The model under review builds one solid part; all positions refer to its coordinate system, in mm. A direction names the side the tool comes from. Round coordinates to 2 decimals unless told otherwise and drop trailing zeros. Loops run counter-clockwise (first coordinate to the right, second up) from the corner with the lowest first, then second, coordinate; pieces in that order, holes last. Notation, with made-up numbers: (3.5, 85.25) - (42.5, 85.25) arc R18 cw to (42.5, 109.25) - close; hole circle Ø3 at (-34, 13). An arc over 180 degrees is marked (long way). Answer as CSV lines item,"result".
from build123d import *

# Parameters (mm, degrees)
SKETCH2_W           = 86.9
SKETCH2_H           = 57
SKETCH2_W_2         = 86.5
SKETCH2_H_2         = 56.6
SKETCH2_W_3         = 75.7
SKETCH2_H_3         = 51.1
BOSS_EXTRUDE2_DEPTH = 1.5
SKETCH2_3_W         = 96.4
SKETCH2_3_H         = 63
SKETCH2_3_W_2       = 86.9
SKETCH2_3_H_2       = 57
BOSS_EXTRUDE3_DEPTH = 27
CHAMFER1_SIZE       = 1
SKETCH3_W           = 96.4
SKETCH3_H           = 63
SKETCH3_W_2         = 93.4
SKETCH3_H_2         = 60
BOSS_EXTRUDE4_DEPTH = 1.5
CHAMFER2_SIZE       = 1.5
SKETCH6_W           = 9.728035046
SKETCH6_H           = 14
CUT_EXTRUDE1_DEPTH  = 6
SKETCH10_W          = 3
SKETCH10_H          = 37.1
CUT_EXTRUDE2_DEPTH  = 23.4
SKETCH11_W          = 3.109966679
SKETCH11_H          = 18.3
CUT_EXTRUDE6_DEPTH  = 20.1
SKETCH12_W          = 13.8
SKETCH12_H          = 3.233091644
CUT_EXTRUDE7_DEPTH  = 10
SKETCH13_W          = 20.000720153
SKETCH13_H          = 4.04568645
CUT_EXTRUDE8_DEPTH  = 14
SKETCH15_W          = 10.8
SKETCH15_H          = 3.606090768
CUT_EXTRUDE9_DEPTH  = 13.4
CHAMFER3_SIZE       = 1.5
CHAMFER4_SIZE       = 1.5
CHAMFER5_SIZE       = 1.5
CHAMFER6_SIZE       = 1.5
CHAMFER7_SIZE       = 1.5
CUT_EXTRUDE11_DEPTH = 4
CUT_EXTRUDE12_DEPTH = 8
SKETCH19_R          = 3.5
CUT_EXTRUDE13_DEPTH = 10
CUT_EXTRUDE14_DEPTH = 4.8


with BuildPart() as part:
    # Sketch2 → Boss-Extrude2 (new body)
    # profile 1 of 2: a face of its own
    with BuildSketch(Plane(origin=(0, 0, 0), x_dir=(0, 0, -1), z_dir=(1, 0, 0))):
        with Locations((-2.142915598, 3.029012225)):
            Rectangle(SKETCH2_W, SKETCH2_H)
        with Locations((-2.142915598, 3.029012225)):
            Rectangle(SKETCH2_W_2, SKETCH2_H_2, mode=Mode.SUBTRACT)
    # profile 2 of 2: a face of its own
    with BuildSketch(Plane(origin=(0, 0, 0), x_dir=(0, 0, -1), z_dir=(1, 0, 0))):
        with Locations((-2.142915598, 3.029012225)):
            Rectangle(SKETCH2_W_2, SKETCH2_H_2)
        with Locations((-0.142915598, 3.279012225)):
            Rectangle(SKETCH2_W_3, SKETCH2_H_3, mode=Mode.SUBTRACT)
    extrude(amount=-BOSS_EXTRUDE2_DEPTH)

    # Sketch2_3 → Boss-Extrude3 (add)
    with BuildSketch(Plane(origin=(0, 0, 0), x_dir=(0, 0, -1), z_dir=(1, 0, 0))):
        with Locations((-0.392915598, 3.029012225)):
            Rectangle(SKETCH2_3_W, SKETCH2_3_H)
        with Locations((-2.142915598, 3.029012225)):
            Rectangle(SKETCH2_3_W_2, SKETCH2_3_H_2, mode=Mode.SUBTRACT)
    extrude(amount=-BOSS_EXTRUDE3_DEPTH)

    # Chamfer1
    chamfer1_edges = [part.edges().sort_by_distance(p)[0] for p in [
        (-0.75, 28.829012225, 37.992915598),
        (-0.75, -22.270987775, 37.992915598),
        (-0.75, -22.270987775, -37.707084402),
        (-0.75, 28.829012225, -37.707084402),
    ]]
    chamfer(chamfer1_edges, length=CHAMFER1_SIZE)

    # Sketch3 → Boss-Extrude4 (add)
    with BuildSketch(Plane.ZY.offset(27)):
        with Locations((0.392915598, 3.029012225)):
            Rectangle(SKETCH3_W, SKETCH3_H)
        with Locations((0.392915598, 3.029012225)):
            Rectangle(SKETCH3_W_2, SKETCH3_H_2, mode=Mode.SUBTRACT)
    extrude(amount=BOSS_EXTRUDE4_DEPTH)

    # Chamfer2
    chamfer2_edges = [part.edges().sort_by_distance(p)[0] for p in [
        (-14.25, 34.529012225, -47.807084402),
        (-14.25, -28.470987775, -47.807084402),
        (-14.25, -28.470987775, 48.592915598),
        (-14.25, 34.529012225, 48.592915598),
    ]]
    chamfer(chamfer2_edges, length=CHAMFER2_SIZE)

    # Sketch6 → Cut-Extrude1 (cut)
    with BuildSketch(Plane.ZY.offset(28.5)):
        with Locations((-46.171101925, 2.829012225)):
            Rectangle(SKETCH6_W, SKETCH6_H)
    extrude(amount=-CUT_EXTRUDE1_DEPTH, mode=Mode.SUBTRACT)

    # Sketch10 → Cut-Extrude2 (cut)
    with BuildSketch(Plane.ZY.offset(28.5)):
        with Locations((47.092915598, -6.920987775)):
            Rectangle(SKETCH10_W, SKETCH10_H)
    extrude(amount=-CUT_EXTRUDE2_DEPTH, mode=Mode.SUBTRACT)

    # Sketch11 → Cut-Extrude6 (cut)
    with BuildSketch(Plane.ZY.offset(28.5)):
        with Locations((47.037932259, 20.779012225)):
            Rectangle(SKETCH11_W, SKETCH11_H)
    extrude(amount=-CUT_EXTRUDE6_DEPTH, mode=Mode.SUBTRACT)

    # Sketch12 → Cut-Extrude7 (cut)
    with BuildSketch(Plane.ZY.offset(28.5)):
        with Locations((-30.410119612, 32.912466403)):
            Rectangle(SKETCH12_W, SKETCH12_H)
    extrude(amount=-CUT_EXTRUDE7_DEPTH, mode=Mode.SUBTRACT)

    # Sketch13 → Cut-Extrude8 (cut)
    with BuildSketch(Plane.ZY.offset(28.5)):
        with Locations((-9.312541512, 33.035392559)):
            Rectangle(SKETCH13_W, SKETCH13_H)
    extrude(amount=-CUT_EXTRUDE8_DEPTH, mode=Mode.SUBTRACT)

    # Sketch15 → Cut-Extrude9 (cut)
    with BuildSketch(Plane.ZY.offset(28.5)):
        with Locations((12.393292701, 33.319062827)):
            Rectangle(SKETCH15_W, SKETCH15_H)
    extrude(amount=-CUT_EXTRUDE9_DEPTH, mode=Mode.SUBTRACT)

    # Chamfer3
    chamfer3_edges = [part.edges().sort_by_distance(p)[0] for p in [
        (-18.5, 33.029012225, -37.310119612),
        (-18.5, 33.029012225, -23.510119612),
    ]]
    chamfer(chamfer3_edges, length=CHAMFER3_SIZE)

    # Chamfer4
    chamfer4_edges = [part.edges().sort_by_distance(p)[0] for p in [
        (-14.5, 33.029012225, -19.312901588),
        (-14.5, 33.029012225, 0.687818565),
    ]]
    chamfer(chamfer4_edges, length=CHAMFER4_SIZE)

    # Chamfer5
    chamfer5_edges = [part.edges().sort_by_distance(p)[0] for p in [
        (-15.1, 33.029012225, 6.993292701),
        (-15.1, 33.029012225, 17.793292701),
    ]]
    chamfer(chamfer5_edges, length=CHAMFER5_SIZE)

    # Chamfer6
    chamfer6_edges = [part.edges().sort_by_distance(p)[0] for p in [
        (-22.5, -4.170987775, -44.557084402),
        (-22.5, 9.829012225, -44.557084402),
    ]]
    chamfer(chamfer6_edges, length=CHAMFER6_SIZE)

    # Chamfer7
    chamfer7_edges = [part.edges().sort_by_distance(p)[0] for p in [
        (-5.1, 11.629012225, 47.092915598),
        (-5.1, -25.470987775, 47.092915598),
    ]]
    chamfer(chamfer7_edges, length=CHAMFER7_SIZE)

    # Sketch17 → Cut-Extrude11 (cut)
    with BuildSketch(Plane.XZ.offset(28.470987775)):
        with BuildLine():
            Line((-20.830033603, 35.662637039), (-7.669966397, 35.662637039))
            ThreePointArc((-7.669966397, 35.662637039), (-6.419966397, 34.412637039), (-7.669966397, 33.162637039))
            Line((-7.669966397, 33.162637039), (-20.830033603, 33.162637039))
            ThreePointArc((-20.830033603, 33.162637039), (-22.080033603, 34.412637039), (-20.830033603, 35.662637039))
        make_face()
        with BuildLine():
            Line((-20.830033603, 29.962637039), (-7.669966397, 29.962637039))
            ThreePointArc((-7.669966397, 29.962637039), (-6.419966397, 28.712637039), (-7.669966397, 27.462637039))
            Line((-7.669966397, 27.462637039), (-20.830033603, 27.462637039))
            ThreePointArc((-20.830033603, 27.462637039), (-22.080033603, 28.712637039), (-20.830033603, 29.962637039))
        make_face()
        with BuildLine():
            Line((-20.830033603, 24.262637039), (-7.669966397, 24.262637039))
            ThreePointArc((-7.669966397, 24.262637039), (-6.419966397, 23.012637039), (-7.669966397, 21.762637039))
            Line((-7.669966397, 21.762637039), (-20.830033603, 21.762637039))
            ThreePointArc((-20.830033603, 21.762637039), (-22.080033603, 23.012637039), (-20.830033603, 24.262637039))
        make_face()
        with BuildLine():
            Line((-20.830033603, 18.562637039), (-7.669966397, 18.562637039))
            ThreePointArc((-7.669966397, 18.562637039), (-6.419966397, 17.312637039), (-7.669966397, 16.062637039))
            Line((-7.669966397, 16.062637039), (-20.830033603, 16.062637039))
            ThreePointArc((-20.830033603, 16.062637039), (-22.080033603, 17.312637039), (-20.830033603, 18.562637039))
        make_face()
        with BuildLine():
            Line((-20.830033603, 12.862637039), (-7.669966397, 12.862637039))
            ThreePointArc((-7.669966397, 12.862637039), (-6.419966397, 11.612637039), (-7.669966397, 10.362637039))
            Line((-7.669966397, 10.362637039), (-20.830033603, 10.362637039))
            ThreePointArc((-20.830033603, 10.362637039), (-22.080033603, 11.612637039), (-20.830033603, 12.862637039))
        make_face()
    extrude(amount=-CUT_EXTRUDE11_DEPTH, mode=Mode.SUBTRACT)

    # Sketch18 → Cut-Extrude12 (cut)
    with BuildSketch(Plane(origin=(0, 0, -47.807084402), x_dir=(-1, 0, 0), z_dir=(0, 0, -1))):
        with BuildLine():
            Line((17, 23.129012225), (17, 5.129012225))
            ThreePointArc((17, 5.129012225), (15.5, 3.629012225), (14, 5.129012225))
            Line((14, 5.129012225), (14, 23.129012225))
            ThreePointArc((14, 23.129012225), (15.5, 24.629012225), (17, 23.129012225))
        make_face()
    extrude(amount=-CUT_EXTRUDE12_DEPTH, mode=Mode.SUBTRACT)

    # Sketch19 → Cut-Extrude13 (cut)
    with BuildSketch(Plane(origin=(0, 0, -47.807084402), x_dir=(-1, 0, 0), z_dir=(0, 0, -1))):
        with Locations(Location((15.5, -16.470987775, 0), (0, 0, 90))):
            Circle(SKETCH19_R)
    extrude(amount=-CUT_EXTRUDE13_DEPTH, mode=Mode.SUBTRACT)

    # Sketch21 → Cut-Extrude14 (cut)
    with BuildSketch(Plane.XY.offset(-41.307084402)):
        Polygon((-15.5, -23.110987775), (-9.749591319, -19.790987775), (-9.749591319, -13.150987775), (-15.5, -9.830987775), (-21.250408681, -13.150987775), (-21.250408681, -19.790987775), align=None)
    extrude(amount=-CUT_EXTRUDE14_DEPTH, mode=Mode.SUBTRACT)


solid = part.part
1. Draft analysis for pull direction Y (two halves, no side actions). For faces 5 (the face through (-8, 11.629, 47)), 6 (the face through (-8.4, 21, 47)), 7 (the face through (-23, 33, 6.993)), 8 (the face through (-14, -28.471, 0)), state which applies: +Y half, -Y half, draft (parallel to the pull), parting line (faces both ways), or undercut.
Numbers:
face 5,"undercut"
face 6,"undercut"
face 7,"draft"
face 8,"-Y half"
2. Take a section at C-C (y = -17.5). State the section outline as (x, z) points.
Numbers:
outline,"(-28.5, -47.81) - (-18.85, -47.81) - (-18.85, -46.11) - (-21.25, -46.11) - (-21.25, -41.31) - (-27, -41.31) - (-27, -46.31) - (-28.5, -46.31) - close; (-12.15, -47.81) - (0, -47.81) - (0, -37.71) - (-1.5, -37.71) - (-1.5, -41.31) - (-9.75, -41.31) - (-9.75, -46.11) - (-12.15, -46.11) - close; (-5.1, 45.59) - (-1.5, 45.59) - (-1.5, 37.99) - (0, 37.99) - (0, 48.59) - (-5.1, 48.59) - close"
3. Take a section at A-A (y = 16). State the section outline as (x, z) points.
Numbers:
outline,"(-28.5, -47.81) - (-17, -47.81) - (-17, -41.31) - (-27, -41.31) - (-27, -46.31) - (-28.5, -46.31) - close; (-14, -47.81) - (0, -47.81) - (0, -37.71) - (-1.5, -37.71) - (-1.5, -41.31) - (-14, -41.31) - close; (-8.4, 45.59) - (-1.5, 45.59) - (-1.5, 37.99) - (0, 37.99) - (0, 48.59) - (-8.4, 48.59) - close"
4. Clearance check with flat-ended pins moving along their axes: pin 1 (0.5 mm diameter, centred on y = 32, z = 4.5, fed in from -X); pin 2 (2 mm diameter, centred on x = -9, y = -8.5, fed in from +Z); pin 3 (3.5 mm diameter, centred on y = -3, z = 47.5, fed in from -X). State where each tip first meets the part, or that it passes through.
Numbers:
pin 1,"stops at x = -27"
pin 2,"stops at z = -41.31"
pin 3,"stops at x = -5.1"
5. Take a section at B-B (x = -3.75). State the section outline as (y, z) points.
Numbers:
outline,"(-28.47, -46.31) - (-26.97, -47.81) - (33.03, -47.81) - (34.53, -46.31) - (34.53, 47.09) - (33.03, 48.59) - (-26.97, 48.59) - (-28.47, 47.09) - close; hole (-25.47, -41.31) - (31.53, -41.31) - (31.53, 45.59) - (-25.47, 45.59) - close"
6. Wall thickness on probe 1 along Z at (x, y) = (-2.75, 20); probe 2 along Y at (x, z) = (-25.75, 36); probe 3 along Z at (x, y) = (-21.5, 14.5): over which ranges is each line inside the solid? List them lowest first.
Numbers:
probe 1,"z = -47.81 to -41.31, 45.59 to 48.59"
probe 2,"y = -28.47 to -25.47, 31.53 to 34.53"
probe 3,"z = -47.81 to -41.31"
7. Tool access review of faces 1 (the face through (-14, 3, -41.307)), 2 (the face through (-14, -27, 10.363)), 3 (the face through (-23, 33, 17.793)), 4 (the face through (-13, -19.3, -46.107)): name each direction out of +Z, -Z, +X, -X, +Y, -Y from which nothing blocks a thin tool from reaching the whole face with its end or side.
Numbers:
face 1,"-X"
face 2,"-Y"
face 3,"-X, +Y"
face 4,"+Z"
